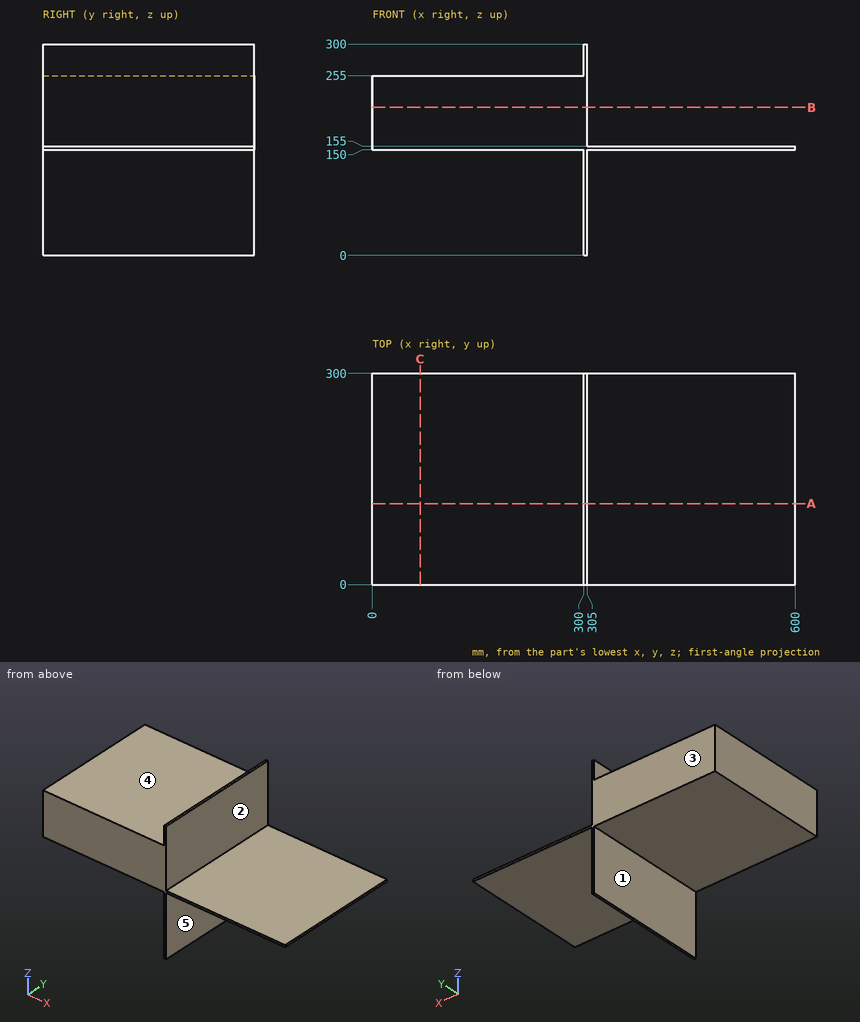
Study the drawing (mm; zero at the part's minimum x, y, z) and answer. A direction names the side the tool comes from. Give positions to 0.01 mm unless a question says otherwise; leave off trailing zeros. Loops run counter-clockwise (first coordinate to the right, second up) from the corner with the lowest first, then second, coordinate; pieces in that order, holes last. Notation, with made-up numbers: M 39.5,-4.75 L 45.5,-4.75 A14 cw 45.5,22.25 Z; hole C -10,5.5 d1. An arc over 180 degrees is marked long. One line per item, written item: value. Start each with the question number.
1. Each of these flat-tipped pins is pushed along its axis until it touches: P1, Ø12, axis at x = 506.5, y = 60.5, coming from the -Z side; P2, Ø2, axis at y = 144.5, z = 252, coming from the +X side; P3, Ø12, axis at x = 335, y = 234, coming from the +Z side. Where does it stop, or does it pass through?
2. Find section C-C (x = 68). Give the vertices of the cut face in (y, z).
3. Find section A-A (y = 115). Give the vertices of the cut face in (x, z), and give its area (3 significant figures).
4. Which of the six approach directions +Z, -Z, +X, -X, +Y, -Y give full straight-line access (tool end or side, diameter ignored) to the marked faces 1, 2, 3, 4 and 5?
5. Find section B-B (z = 210). Give the vertices of the cut face in (x, y), and give its area (3 significant figures).
6. Find the intervals of material crossed by probe 1 along X at (y, z) = (121.5, 107.5); probe 2 along Z at (x, y) = (98.5, 287.5); probe 3 along Z at (x, y) = (521, 223.5), in increasing order.
Reported:
1. P1: stops at z = 150
1. P2: stops at x = 305
1. P3: stops at z = 155
2. outline: M 0,150 L 300,150 L 300,255 L 0,255 Z
3. outline: M 0,150 L 300,150 L 300,0 L 305,0 L 305,150 L 600,150 L 600,155 L 305,155 L 305,300 L 300,300 L 300,255 L 0,255 Z
3. area: 34,500 mm²
4. face 1: -Z, -X, +Y, -Y
4. face 2: +Z, +X, +Y, -Y
4. face 3: +Z, -Z, +X, -X, +Y
4. face 4: +Z, -X, +Y, -Y
4. face 5: -Z, +X, +Y, -Y
5. outline: M 0,0 L 305,0 L 305,300 L 0,300 Z
5. area: 91,500 mm²
6. probe 1: x = 300 to 305
6. probe 2: z = 150 to 255
6. probe 3: z = 150 to 155
